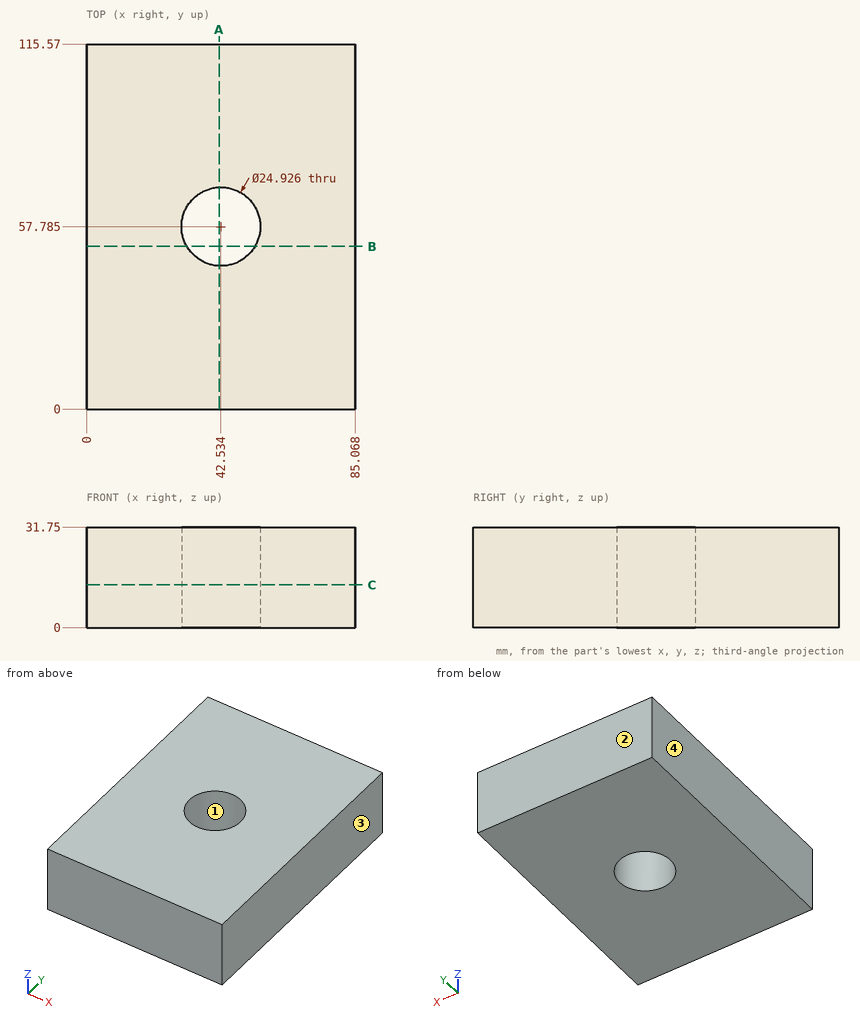
Source: three-view drawing plus pictorial views. Frame: mm from the lowest corner of the part. Give positions to 0.01 mm unless a question says otherwise; leave off trailing zeros. Loops run counter-clockwise (first coordinate to the right, second up) from the corner with the lowest first, then second, coordinate; pieces in that order, holes last. Notation, with made-up numbers: (18, 58.25) -> (60, 58.25) arc R25 ccw to (60, 93.25) -> close; hole circle Ø4 at (48.25, 51). An arc over 180 degrees is marked (long way). Put each result on its own line as item: value. Start each with the question number.
1) Draft query along X for the marked faces 1, 2, 3 and 4. Return one class per face: released by +X, released by -X, zero draft, split by the parting line, or undercut.
2) Cut plane C-C (z = 13.5). Return loops of the section in (x, y) (1 decimal).
3) Cut plane A-A (x = 42). Return loops of the section in (y, z).
4) Material intervals for probe 1 along X at (y, z) = (55, 24) (1 decimal); probe 2 along X at (y, z) = (49, 20) (1 decimal); probe 3 along Y at (x, z) = (44.5, 30), sorted ascending.
5) Cut plane B-B (y = 51.5). Return loops of the section in (x, z).
Results are:
1. face 1: undercut
1. face 2: zero draft
1. face 3: released by +X
1. face 4: released by -X
2. outline: (0, 0) -> (85.1, 0) -> (85.1, 115.6) -> (0, 115.6) -> close; hole circle Ø24.9 at (42.5, 57.8)
3. outline: (0, 0) -> (45.33, 0) -> (45.33, 31.75) -> (0, 31.75) -> close; (70.24, 0) -> (115.57, 0) -> (115.57, 31.75) -> (70.24, 31.75) -> close
4. probe 1: x = 0 to 30.4, 54.7 to 85.1
4. probe 2: x = 0 to 33.7, 51.4 to 85.1
4. probe 3: y = 0 to 45.48, 70.09 to 115.57
5. outline: (0, 0) -> (31.77, 0) -> (31.77, 31.75) -> (0, 31.75) -> close; (53.3, 0) -> (85.07, 0) -> (85.07, 31.75) -> (53.3, 31.75) -> close
